Read the model definition and answer for the solid it produces. Units are mm, in the model's axes. Face numbers are marked on the shaded views. Give positions to 0.01 mm unless a question says otherwise; leave off trailing zeros. Write each loop counter-clockwise with the first axis right and the second up, starting at its lowest first coordinate (ties: lowest second). Pieces come first, ordered by that corner, then holes. Notation, with made-up numbers: M -3,71 L 11,71 A8 cw 11,82 Z; hole C 80,-23.5 d5. An arc over 180 degrees is marked long. Put each result on its own line as item: value.
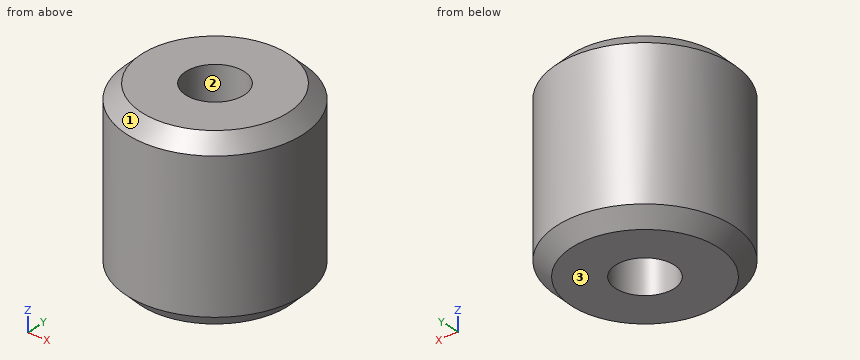
from build123d import *

# Parameters (mm, degrees)
SKETCH1_R           = 6
BOSS_EXTRUDE1_DEPTH = 12
SKETCH2_R           = 2
CUT_EXTRUDE1_DEPTH  = 13
CHAMFER1_SIZE       = 1


with BuildPart() as part:
    # Sketch1 → Boss-Extrude1 (new body)
    with BuildSketch(Plane.XY):
        Circle(SKETCH1_R)
    extrude(amount=BOSS_EXTRUDE1_DEPTH)

    # Sketch2 → Cut-Extrude1 (cut, through all)
    with BuildSketch(Plane.XY):
        Circle(SKETCH2_R)
    extrude(amount=CUT_EXTRUDE1_DEPTH, mode=Mode.SUBTRACT)

    # Chamfer1
    chamfer1_edges = [part.edges().sort_by_distance(p)[0] for p in [
        (-6, 0, 0),
        (-6, 0, 12),
    ]]
    chamfer(chamfer1_edges, length=CHAMFER1_SIZE)


solid = part.part
(1) Section A-A on y = 0 is taken. Determine the outline of the cut face in (x, z).
Result:
outline: M -6,1 L -5,0 L -2,0 L -2,12 L -5,12 L -6,11 Z; M 2,0 L 5,0 L 6,1 L 6,11 L 5,12 L 2,12 Z
(2) Straight lines are drawn through the part: line 1 along Y through (x, z) = (0, 5.5); line 2 along Y through (x, z) = (0.5, 3.25); line 3 along Z through (x, y) = (3.5, 4.75). For each, find the intervals that lie inside material, in ascending order. Write a range as from..to.
Result:
line 1: y = -6..-2, 2..6
line 2: y = -5.98..-1.94, 1.94..5.98
line 3: z = 0.9..11.1
(3) Given pin 1 Ø1.5 at (y, z) = (3.5, 10.5) entering from -X; pin 2 Ø5 at (x, z) = (4, 7) entering from +Y; pin 3 Ø3 at (x, z) = (4.5, 4) entering from +Y, each flat-ended and moving along its own axis, determine where each tip first touches the part or whether it passes through.
Result:
pin 1: stops at x = -5.33
pin 2: stops at y = 5.81
pin 3: stops at y = 5.2
(4) For a pull along Y with two mould halves and no side action, classify the marked faces 1, 2 and 3 as +Y half, -Y half, draft (parallel to the pull), parting line (faces both ways), or undercut.
Result:
face 1: parting line
face 2: undercut
face 3: draft
(5) Section C-C on z = 5 is taken. Determine the outline of the cut face in (x, y), and give its area (3 significant figures).
Result:
outline: C 0,0 d12; hole C 0,0 d4
area: 101 mm²
